from build123d import *

# Parameters (mm, degrees)
SKETCH1_W      = 65
SKETCH1_H      = 40
EXTRUDE1_DEPTH = 14
SKETCH2_R      = 3.5
EXTRUDE2_DEPTH = 41


with BuildPart() as part:
    # Sketch1 → Extrude1 (new body)
    with BuildSketch(Plane.XY):
        with Locations((32.5, 20)):
            Rectangle(SKETCH1_W, SKETCH1_H)
    extrude(amount=EXTRUDE1_DEPTH)

    # Sketch2 → Extrude2 (cut, through all)
    with BuildSketch(Plane(origin=(0, 40, 0), x_dir=(1, 0, 0), z_dir=(0, 1, 0))):
        with Locations(Location((8.75, -7, 0), (0, 0, 270))):  # turned: the seam where the file's is
            Circle(SKETCH2_R)
        with Locations(Location((56.25, -7, 0), (0, 0, 270))):  # turned: the seam where the file's is
            Circle(SKETCH2_R)
    extrude(amount=-EXTRUDE2_DEPTH, mode=Mode.SUBTRACT)


solid = part.part
Here's how the part is built. I have some questions about the finished solid (model axes, mm). Coordinates: 2 decimals unless noted, no trailing zeros. Write each loop counter-clockwise with the first axis right and the second up, starting at its lowest first coordinate (ties: lowest second). Pieces come first, ordered by that corner, then holes. Notation, with made-up numbers: (70, -32) - (95, -32) arc R15 ccw to (95, -24) - close; hole circle Ø7 at (-26.75, -7). An arc over 180 degrees is marked (long way). Use one line per item in the form item = value.
1) Suppose I cut it at B-B, the plane z = 7. Write out the boundary of the cut face in (x, y).
Solved:
outline = (0, 0) - (5.25, 0) - (5.25, 40) - (0, 40) - close; (12.25, 0) - (52.75, 0) - (52.75, 40) - (12.25, 40) - close; (59.75, 0) - (65, 0) - (65, 40) - (59.75, 40) - close
2) I'm going to push a flat-ended pin straight in: P1, Ø2, axis at x = 42.5, y = 29, coming from the -Z side. Where does the tip first touch, or does it pass through?
Solved:
P1 = 0
3) Thinking about a two-plate mould opening in X: for faces 1 (the cylindrical face through (54.12, 20.28, 4.223)), 2 (the flat face through (32, 40, 7)), 3 (the flat face through (0, 20, 7)), 4 (the cylindrical face through (5.333, 20.28, 6.241)), which applies, released by +X, released by -X, zero draft, split by the parting line, or undercut?
Solved:
face_1 = undercut
face_2 = zero draft
face_3 = released by -X
face_4 = undercut
4) Suppose I cut it at C-C, the plane y = 15. Write out the boundary of the cut face in (x, z), plus the area to 3 significant figures.
Solved:
outline = (0, 0) - (65, 0) - (65, 14) - (0, 14) - close; hole circle Ø7 at (8.75, 7); hole circle Ø7 at (56.25, 7)
area = 833 mm2
5) I need wall thicknesses on line 1 (X direction, y = 28.5, z = 7); line 2 (X direction, y = 22.5, z = 5); line 3 (Z direction, x = 8, y = 25). Which ranges of each line are inside material? Lowest first, please.
Solved:
line_1 = 0 to 5.25, 12.25 to 52.75, 59.75 to 65
line_2 = 0 to 5.88, 11.62 to 53.38, 59.12 to 65
line_3 = 0 to 3.58, 10.42 to 14
6) Suppose I cut it at A-A, the plane x = 56.25. Write out the boundary of the cut face in (y, z).
Solved:
outline = (0, 0) - (40, 0) - (40, 3.5) - (0, 3.5) - close; (0, 10.5) - (40, 10.5) - (40, 14) - (0, 14) - close
